from build123d import *

# Parameters (mm, degrees)
CROQUIS2_R              = 1.5875
CROQUIS2_R_2            = 1.59
CROQUIS2_W              = 2.5
CROQUIS2_H              = 4.5
SALIENTE_EXTRUIR1_DEPTH = 2


with BuildPart() as part:
    # Croquis2 → Saliente-Extruir1 (new body)
    with BuildSketch(Plane(origin=(0, 0, 0), x_dir=(1, 0, 0), z_dir=(0, 1, 0))):
        with BuildLine():
            ThreePointArc((-15.794895255, -5.504961381), (-16.432835447, -9.019479294), (-18.265262487, -12.08558676))
            Line((-18.265262487, -12.08558676), (-25.665833323, -20.55341124))
            ThreePointArc((-25.665833323, -20.55341124), (-26.522572581, -23.091497469), (-25.333680736, -25.492001591))
            Line((-25.333680736, -25.492001591), (-21.870049663, -28.519089265))
            ThreePointArc((-21.870049663, -28.519089265), (-19.331963434, -29.375828523), (-16.931459311, -28.186936679))
            Line((-16.931459311, -28.186936679), (-10.339710555, -20.824046432))
            ThreePointArc((-10.339710555, -20.824046432), (-6.969614061, -18.364525857), (-2.889258582, -17.494186265))
            Line((-2.889258582, -17.494186265), (2.889258582, -17.494186265))
            ThreePointArc((2.889258582, -17.494186265), (6.969614061, -18.364525857), (10.339710555, -20.824046432))
            Line((10.339710555, -20.824046432), (16.931459311, -28.186936679))
            ThreePointArc((16.931459311, -28.186936679), (19.331963434, -29.375828523), (21.870049663, -28.519089265))
            Line((21.870049663, -28.519089265), (25.333680736, -25.492001591))
            ThreePointArc((25.333680736, -25.492001591), (26.522572581, -23.091497469), (25.665833323, -20.55341124))
            Line((25.665833323, -20.55341124), (18.265262487, -12.08558676))
            ThreePointArc((18.265262487, -12.08558676), (16.432835447, -9.019479294), (15.794895255, -5.504961381))
            Line((15.794895255, -5.504961381), (15.794895255, 5.504961381))
            ThreePointArc((15.794895255, 5.504961381), (16.432835447, 9.019479294), (18.265262487, 12.08558676))
            Line((18.265262487, 12.08558676), (25.665833323, 20.55341124))
            ThreePointArc((25.665833323, 20.55341124), (26.522572581, 23.091497469), (25.333680736, 25.492001591))
            Line((25.333680736, 25.492001591), (21.870049663, 28.519089265))
            Line((21.870049663, 28.519089265), (19.624131665, 30.812041893))
            Line((19.624131665, 30.812041893), (17.831541391, 35.250897727))
            ThreePointArc((17.831541391, 35.250897727), (15.348771565, 36.809322612), (13.092386176, 34.938077274))
            Line((13.092386176, 34.938077274), (10.747335089, 25.829720308))
            Line((10.747335089, 25.829720308), (10.537909559, 25.016295609))
            ThreePointArc((10.537909559, 25.016295609), (9.494618305, 22.668322934), (7.742465325, 20.789123037))
            Line((7.742465325, 20.789123037), (2.462782312, 30.427383086))
            ThreePointArc((2.462782312, 30.427383086), (1.432591067, 31.523244144), (0, 31.981379817))
            ThreePointArc((0, 31.981379817), (-1.432591067, 31.523244144), (-2.462782312, 30.427383086))
            Line((-2.462782312, 30.427383086), (-7.742465325, 20.789123037))
            ThreePointArc((-7.742465325, 20.789123037), (-9.494618305, 22.668322934), (-10.537909559, 25.016295609))
            Line((-10.537909559, 25.016295609), (-13.092386176, 34.938077274))
            ThreePointArc((-13.092386176, 34.938077274), (-15.348771565, 36.809322612), (-17.831541391, 35.250897727))
            Line((-17.831541391, 35.250897727), (-19.624131665, 30.812041893))
            Line((-19.624131665, 30.812041893), (-21.870049663, 28.519089265))
            Line((-21.870049663, 28.519089265), (-23.601865199, 27.005545428))
            Line((-23.601865199, 27.005545428), (-25.333680736, 25.492001591))
            ThreePointArc((-25.333680736, 25.492001591), (-26.522572581, 23.091497469), (-25.665833323, 20.55341124))
            Line((-25.665833323, 20.55341124), (-18.265262487, 12.08558676))
            ThreePointArc((-18.265262487, 12.08558676), (-16.432835447, 9.019479294), (-15.794895255, 5.504961381))
            Line((-15.794895255, 5.504961381), (-15.794895255, -5.504961381))
        make_face()
        with Locations(Location((-21.166889821, -24.21941655, 0), (0, 0, 270))):
            Circle(CROQUIS2_R, mode=Mode.SUBTRACT)
        with Locations(Location((-15.25, -15.25, 0), (0, 0, 270))):
            Circle(CROQUIS2_R_2, mode=Mode.SUBTRACT)
        with BuildLine():
            Line((-8.099892262, -2.037172726), (-8.099892262, -4.090589628))
            ThreePointArc((-8.099892262, -4.090589628), (-9.349892262, -5.340589628), (-10.599892262, -4.090589628))
            Line((-10.599892262, -4.090589628), (-10.599892262, -2.037172726))
            ThreePointArc((-10.599892262, -2.037172726), (-9.349892262, -0.787172726), (-8.099892262, -2.037172726))
        make_face(mode=Mode.SUBTRACT)
        with BuildLine():
            ThreePointArc((-10.599892262, 4.090589628), (-9.349892262, 5.340589628), (-8.099892262, 4.090589628))
            Line((-8.099892262, 4.090589628), (-8.099892262, 2.037172726))
            ThreePointArc((-8.099892262, 2.037172726), (-9.349892262, 0.787172726), (-10.599892262, 2.037172726))
            Line((-10.599892262, 2.037172726), (-10.599892262, 4.090589628))
        make_face(mode=Mode.SUBTRACT)
        with BuildLine():
            Line((-3.387203965, -1.942277199), (-3.387203965, -2.839990658))
            ThreePointArc((-3.387203965, -2.839990658), (-4.637203965, -4.089990658), (-5.887203965, -2.839990658))
            Line((-5.887203965, -2.839990658), (-5.887203965, -1.942277199))
            ThreePointArc((-5.887203965, -1.942277199), (-4.637203965, -0.692277199), (-3.387203965, -1.942277199))
        make_face(mode=Mode.SUBTRACT)
        with BuildLine():
            ThreePointArc((-5.887203965, 2.839990658), (-4.637203965, 4.089990658), (-3.387203965, 2.839990658))
            Line((-3.387203965, 2.839990658), (-3.387203965, 1.942277199))
            ThreePointArc((-3.387203965, 1.942277199), (-4.637203965, 0.692277199), (-5.887203965, 1.942277199))
            Line((-5.887203965, 1.942277199), (-5.887203965, 2.839990658))
        make_face(mode=Mode.SUBTRACT)
        with Locations(Location((21.166889821, -24.21941655, 0), (0, 0, 270))):
            Circle(CROQUIS2_R, mode=Mode.SUBTRACT)
        with Locations(Location((15.25, -15.25, 0), (0, 0, 270))):
            Circle(CROQUIS2_R_2, mode=Mode.SUBTRACT)
        with BuildLine():
            ThreePointArc((1.25, -5.653716791), (0, -6.903716791), (-1.25, -5.653716791))
            Line((-1.25, -5.653716791), (-1.25, -3.063881177))
            ThreePointArc((-1.25, -3.063881177), (0, -1.813881177), (1.25, -3.063881177))
            Line((1.25, -3.063881177), (1.25, -5.653716791))
        make_face(mode=Mode.SUBTRACT)
        with BuildLine():
            ThreePointArc((5.887203965, -2.839990658), (4.637203965, -4.089990658), (3.387203965, -2.839990658))
            Line((3.387203965, -2.839990658), (3.387203965, -1.942277199))
            ThreePointArc((3.387203965, -1.942277199), (4.637203965, -0.692277199), (5.887203965, -1.942277199))
            Line((5.887203965, -1.942277199), (5.887203965, -2.839990658))
        make_face(mode=Mode.SUBTRACT)
        with BuildLine():
            Line((3.387203965, 1.942277199), (3.387203965, 2.839990658))
            ThreePointArc((3.387203965, 2.839990658), (4.637203965, 4.089990658), (5.887203965, 2.839990658))
            Line((5.887203965, 2.839990658), (5.887203965, 1.942277199))
            ThreePointArc((5.887203965, 1.942277199), (4.637203965, 0.692277199), (3.387203965, 1.942277199))
        make_face(mode=Mode.SUBTRACT)
        with BuildLine():
            ThreePointArc((10.599892262, -4.090589628), (9.349892262, -5.340589628), (8.099892262, -4.090589628))
            Line((8.099892262, -4.090589628), (8.099892262, -2.037172726))
            ThreePointArc((8.099892262, -2.037172726), (9.349892262, -0.787172726), (10.599892262, -2.037172726))
            Line((10.599892262, -2.037172726), (10.599892262, -4.090589628))
        make_face(mode=Mode.SUBTRACT)
        with BuildLine():
            Line((8.099892262, 2.037172726), (8.099892262, 4.090589628))
            ThreePointArc((8.099892262, 4.090589628), (9.349892262, 5.340589628), (10.599892262, 4.090589628))
            Line((10.599892262, 4.090589628), (10.599892262, 2.037172726))
            ThreePointArc((10.599892262, 2.037172726), (9.349892262, 0.787172726), (8.099892262, 2.037172726))
        make_face(mode=Mode.SUBTRACT)
        with Locations(Location((-15.25, 15.25, 0), (0, 0, 270))):
            Circle(CROQUIS2_R_2, mode=Mode.SUBTRACT)
        with BuildLine():
            ThreePointArc((-19.579389821, 24.21941655), (-21.823295119, 22.773979477), (-22.211564099, 25.414745752))
            ThreePointArc((-22.211564099, 25.414745752), (-20.510484522, 25.664853624), (-19.579389821, 24.21941655))
        make_face(mode=Mode.SUBTRACT)
        with Locations((-15.25, 31.000541934)):
            Rectangle(CROQUIS2_W, CROQUIS2_H, mode=Mode.SUBTRACT)
        with BuildLine():
            Line((-1.25, 3.063881177), (-1.25, 5.653716791))
            ThreePointArc((-1.25, 5.653716791), (0, 6.903716791), (1.25, 5.653716791))
            Line((1.25, 5.653716791), (1.25, 3.063881177))
            ThreePointArc((1.25, 3.063881177), (0, 1.813881177), (-1.25, 3.063881177))
        make_face(mode=Mode.SUBTRACT)
        with Locations(Location((15.25, 15.25, 0), (0, 0, 270))):
            Circle(CROQUIS2_R_2, mode=Mode.SUBTRACT)
        with BuildLine():
            ThreePointArc((3.999695887, 15.899705615), (3.300253998, 13.504573342), (1.031076217, 12.466927083))
            Line((1.031076217, 12.466927083), (-1.031076217, 12.466927083))
            ThreePointArc((-1.031076217, 12.466927083), (-3.300253998, 13.504573342), (-3.999695887, 15.899705615))
            Line((-3.999695887, 15.899705615), (-2.500174028, 26.185590314))
            ThreePointArc((-2.500174028, 26.185590314), (0, 28.347706433), (2.500174028, 26.185590314))
            Line((2.500174028, 26.185590314), (3.999695887, 15.899705615))
        make_face(mode=Mode.SUBTRACT)
        with Locations(Location((21.166889821, 24.21941655, 0), (0, 0, 270))):
            Circle(CROQUIS2_R, mode=Mode.SUBTRACT)
        with Locations((15.25, 31.000541934)):
            Rectangle(CROQUIS2_W, CROQUIS2_H, mode=Mode.SUBTRACT)
    extrude(amount=SALIENTE_EXTRUIR1_DEPTH)


solid = part.part
Geometry check sheet. Reference: the model listing, model coordinates, mm. A direction names the side the tool comes from. Give positions to 0.01 mm unless a question says otherwise; leave off trailing zeros. Loops run counter-clockwise (first coordinate to the right, second up) from the corner with the lowest first, then second, coordinate; pieces in that order, holes last.
(1) Section check B-B on z = -19.5. Record the cut outline in (x, y).
From the geometry:
outline: (-24.75, 0) - (-3.47, 0) - (-3.47, 2) - (-24.75, 2) - close; (3.47, 0) - (24.75, 0) - (24.75, 2) - (3.47, 2) - close
(2) Release check for a two-part mould opening along Z. For faces 5 (the flat face through (6, 2, -4)), 6 (the cylindrical face through (-4.66, 0.99, -4.09)), 7 (the cylindrical face through (1.45, 0.99, -31.51)) record: released by +Z, released by -Z, zero draft, split by the parting line, or undercut.
From the geometry:
face 5: zero draft
face 6: undercut
face 7: released by -Z
(3) Section check D-D on z = 0. Record the cut outline in (x, y), then the cut area to 3 significant figures.
From the geometry:
outline: (-15.79, 0) - (15.79, 0) - (15.79, 2) - (-15.79, 2) - close
area: 63.2 mm2
(4) Thickness scan on L1, parallel to X at y = 0.6, z = 5.5; L2, parallel to X at y = 0.65, z = -30; L3, parallel to X at y = 1.35, z = -15.25. Record the ranges inside material, lowest first.
From the geometry:
L1: x = -15.79 to -1.25, 1.25 to 15.79
L2: x = -20.42 to -16.5, -14 to -11.82, -2.7 to 2.7, 11.82 to 14, 16.5 to 20.42
L3: x = -21.03 to -16.84, -13.66 to -4.02, 4.02 to 13.66, 16.84 to 21.03
(5) Section check C-C on y = 1.2. Count the separate pieces of the cut face and the enclosed holes in it, then the cut area to 3 significant figures.
From the geometry:
separate pieces: 1
enclosed holes: 21
area: 1,850 mm2
(6) Section check A-A on z = 15.25. Record the cut outline in (x, y), then the cut area to 3 significant figures.
From the geometry:
outline: (-21.03, 0) - (-16.84, 0) - (-16.84, 2) - (-21.03, 2) - close; (-13.66, 0) - (13.66, 0) - (13.66, 2) - (-13.66, 2) - close; (16.84, 0) - (21.03, 0) - (21.03, 2) - (16.84, 2) - close
area: 71.4 mm2
(7) Set-up check for faces 1 (the flat face through (15, 1, -28.751)), 2 (the cylindrical face through (16.415, 0.986, -8.972)), 3 (the flat face through (-5.066, 0.986, -25.676)), 4 (the cylindrical face through (-16.45, 0.99, -9.07)): record each of +Z, -Z, +X, -X, +Y, -Y from which the full face is reachable in a straight line by a thin tool's end or side.
From the geometry:
face 1: +Y, -Y
face 2: +X, +Y, -Y
face 3: -Z, +Y, -Y
face 4: -X, +Y, -Y
(8) Depth check by flat-ended pin: pin 1 Ø1 at (y, z) = (1.5, -1) entering from +X; pin 2 Ø2.5 at (x, z) = (15.25, 15.25) entering from +Y; pin 3 Ø0.6 at (x, y) = (0, 1) entering from -Z. Enter the tip coordinate at first touch or a pass-through.
From the geometry:
pin 1: stops at x = 15.79
pin 2: passes through
pin 3: stops at z = -31.98
